Model file for the job. Use its own axes, mm. A direction names the side the tool comes from. Round coordinates to 2 decimals unless told otherwise and drop trailing zeros. Loops run counter-clockwise (first coordinate to the right, second up) from the corner with the lowest first, then second, coordinate; pieces in that order, holes last. Notation, with made-up numbers: (3, -37.75) -> (32, -37.75) arc R14 cw to (32, -24.75) -> close; hole circle Ø1 at (74.5, -35.75). An arc over 180 degrees is marked (long way). Use a Markdown table: item, result.
from build123d import *

# Parameters (mm, degrees)
EXTRUDE_1_DEPTH     = 3.5
SKETCH_2_W          = 3.2
SKETCH_2_H          = 3.2
CUT_EXTRUDE_1_DEPTH = 3


with BuildPart() as part:
    # 草图1 → 凸台-拉伸1 (new, symmetric)
    with BuildSketch(Plane.XY):
        Polygon((0, 0), (10, 0), (10, 3), (5, 3), (5, 5), (0, 5), align=None)
    extrude(amount=EXTRUDE_1_DEPTH, both=True)

    # 草图2 → 切除-拉伸1 (cut)
    with BuildSketch(Plane.ZY):
        with Locations((0, 2.5)):
            Rectangle(SKETCH_2_W, SKETCH_2_H)
    extrude(amount=-CUT_EXTRUDE_1_DEPTH, mode=Mode.SUBTRACT)


solid = part.part
Q1. Band-saw the part on B-B, the plane y = 3.65. Give the cut face in (x, z), plus the area to 3 significant figures.
Results list:
| item | result |
|---|---|
| outline | (0, -3.5) -> (5, -3.5) -> (5, 3.5) -> (0, 3.5) -> (0, 1.6) -> (3, 1.6) -> (3, -1.6) -> (0, -1.6) -> close |
| area | 25.4 mm² |
Q2. Band-saw the part on D-D, the plane y = 2.05. Give the cut face in (x, z).
Results list:
| item | result |
|---|---|
| outline | (0, -3.5) -> (10, -3.5) -> (10, 3.5) -> (0, 3.5) -> (0, 1.6) -> (3, 1.6) -> (3, -1.6) -> (0, -1.6) -> close |
Q3. Pull direction Y, two halves, no side cores. Call faces 1 (the face through (1, 2, 1.6)), 2 (the face through (5, 4, 0)), 3 (the face through (3, 5, 0)), 4 (the face through (5, 0, 0)): released by +Y, released by -Y, zero draft, split by the parting line, or undercut.
Results list:
| item | result |
|---|---|
| face 1 | undercut |
| face 2 | zero draft |
| face 3 | released by +Y |
| face 4 | released by -Y |
Q4. Band-saw the part on C-C, the plane x = 2.75. Give the cut face in (y, z), plus the area to 3 significant figures.
Results list:
| item | result |
|---|---|
| outline | (0, -3.5) -> (5, -3.5) -> (5, 3.5) -> (0, 3.5) -> close; hole (0.9, -1.6) -> (4.1, -1.6) -> (4.1, 1.6) -> (0.9, 1.6) -> close |
| area | 24.8 mm² |
Q5. Band-saw the part on A-A, the plane z = -1.25. Give the cut face in (x, y), plus the area to 3 significant figures.
Results list:
| item | result |
|---|---|
| outline | (0, 0) -> (10, 0) -> (10, 3) -> (5, 3) -> (5, 5) -> (0, 5) -> (0, 4.1) -> (3, 4.1) -> (3, 0.9) -> (0, 0.9) -> close |
| area | 30.4 mm² |
Q6. Flat gauge pins, fed straight in: pin 1 (0.6 mm diameter, centred on y = 4.5, z = -0.5, fed in from +X); pin 2 (1 mm diameter, centred on x = 6, z = 0.5, fed in from +Y). Where does each tip first touch, or does it go through?
Results list:
| item | result |
|---|---|
| pin 1 | stops at x = 5 |
| pin 2 | stops at y = 3 |
Q7. Drill centre lines: L1, parallel to Z at x = 1, y = 2.95; L2, parallel to Y at x = 1.5, z = -1.25; L3, parallel to Y at x = 8.5, z = -2.25. Where is each one in solid material? Low to high. Write a range as from..to.
Results list:
| item | result |
|---|---|
| L1 | z = -3.5..-1.6, 1.6..3.5 |
| L2 | y = 0..0.9, 4.1..5 |
| L3 | y = 0..3 |
Q8. Tool access for faces 5 (the face through (4, 2, -3.5)), 6 (the face through (8, 3, 0)), 7 (the face through (1, 4.1, 0)): list every direction of +Z, -Z, +X, -X, +Y, -Y with a clear straight run to the whole face (end or side of a thin tool).
Results list:
| item | result |
|---|---|
| face 5 | -Z, +X, -X, +Y, -Y |
| face 6 | +Z, -Z, +X, +Y |
| face 7 | -X |
